Here's the drawing with two shaded views (mm, measured from the low corner). I have some questions. Round coordinates to 2 decimals unless told otherwise and drop trailing zeros. Write each loop counter-clockwise with the first axis right and the second up, starting at its lowest first coordinate (ties: lowest second). Pieces come first, ordered by that corner, then holes. Notation, with made-up numbers: (-13, 44.5) - (13, 44.5) arc R22 ccw to (13, 56.5) - close; hole circle Ø1 at (70, 8). An arc over 180 degrees is marked (long way). Return JSON: item names as keys, results as strings. Group by question number.
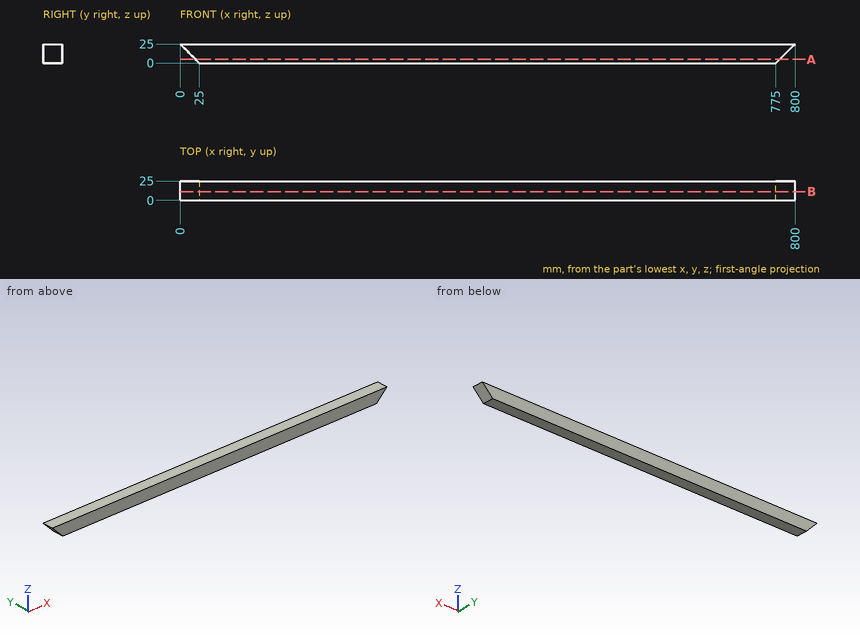
1) Imagine slicing it at B-B (y = 11.5). Please give me the cut outline in (x, z), plus the area to 3 significant figures.
2) I need wall thicknesses on line 1 along X through (y, z) = (22.75, 17); line 2 along X through (y, z) = (10, 17.5). Which ranges of each line are inside material? Lowest first, please.
3) Imagine slicing it at A-A (z = 5). Please give me the cut outline in (x, y), plus the area to 3 significant figures.
4) Will this pin go through, and if not, where does the flat tip stop? pin 1 Ø6 at (y, z) = (12, 21) entering from +X.
Results found:
{
 "1": {"outline": "(0, 25) - (25, 0) - (775, 0) - (800, 25) - close", "area": "19,400 mm²"},
 "2": {"line 1": "x = 8 to 792", "line 2": "x = 7.5 to 792.5"},
 "3": {"outline": "(20, 0) - (780, 0) - (780, 25) - (20, 25) - close", "area": "19,000 mm²"},
 "4": {"pin 1": "stops at x = 799"}
}
